For this review, take the finished solid that the model builds, in its own axes (mm). A direction names the side the tool comes from. Round coordinates to 2 decimals unless told otherwise and drop trailing zeros. Loops run counter-clockwise (first coordinate to the right, second up) from the corner with the lowest first, then second, coordinate; pieces in that order, holes last.
1. Clearance check with flat-ended pins moving along their axes: pin 1 Ø2 at (x, z) = (-67, 3.5) entering from +Y (3 decimals); pin 2 Ø0.8 at (x, z) = (-26.5, -7) entering from +Y; pin 3 Ø4 at (x, z) = (-44.5, 1.5) entering from -Y (3 decimals). State where each tip first meets the part, or that it passes through.
2. Tool access review of faces 4 (the flat face through (-65.25, -1, 1)), 5 (the flat face through (-53.7, -6.405, 6.7)), 6 (the flat face through (-29, -0.89, 5)): name each direction out of +Z, -Z, +X, -X, +Y, -Y from which nothing blocks a thin tool from reaching the whole face with its end or side.
3. Consider section A-A on x = -47. State the section outline as (y, z) points (3 decimals).
4. To check wall thickness, follow line 1 along X through (y, z) = (2.75, 0.5); line 2 along Z through (x, y) = (-40, -4.75); line 3 along Y through (x, z) = (-26.75, -6.9) (3 decimals). State the ranges of each line that lie inside material, in increasing order.
5. Consider section B-B on x = -59. State the section outline as (y, z) points (3 decimals).
6. Draft analysis for pull direction Z (two halves, no side actions). For faces 1 (the cylindrical face through (-73.087, -2.827, 6.014)), 2 (the flat face through (-29, 2, -6)), 3 (the flat face through (-70, 0, 5)), state which applies: released by +Z, released by -Z, zero draft, split by the parting line, or undercut.
Autodesk Inventor part; units mm, degrees
ref_plane "YZ Plane" through (0, 0, 0) normal (1, 0, 0) x (0, 1, 0)
ref_plane "XZ Plane" through (0, 0, 0) normal (0, 1, 0) x (-1, 0, 0)
ref_plane "XY Plane" through (0, 0, 0) normal (0, 0, 1) x (1, 0, 0)
ref_plane "Work Plane1" through (-21.75, 2.25, -0.6) normal (0, 0, 1) x (-1, 0, 0)
ref_plane "Work Plane2" through (-30.217, -5.375, 6) normal (0, 0, 1) x (1, 0, 0)
sketch "Sketch1" plane through (-30.217, -5.375, 6) normal (0, 0, 1) x (1, 0, 0)
  circle A0 centre (2.6155, -1.0303) radius 1.1
  circle A1 centre (3.467, 10) radius 1.5
  line L0 (4.6155, -1.0303) -> (5.967, 8)
  line L1 (0.6155, -1.0303) -> (-44.3845, -1.0303)
  arc A2 (0.6155, -1.0303) -> (4.6155, -1.0303) centre (2.6155, -1.0303) ccw
  line L2 (5.967, 8) -> (5.967, 10)
  line L3 (0.967, 10) -> (-44.033, 10)
  arc A3 (5.967, 10) -> (0.967, 10) centre (3.467, 10) ccw
  line L4 (-44.033, 10) -> (-44.3845, -1.0303)
  point P0 (30.217, 5.375)
  dimension "d0" = 2
  dimension "d1" = 2
  dimension "d2" = 2
  dimension "d3" = 2.5
  dimension "d4" = 2
  dimension "d5" = 2.5
  dimension "d6" = 2.5
  dimension "d7" = 45
  dimension "d8" = 45
extrude "Extrusion1" add sketch "Sketch1" along normal blind 1
sketch "Sketch2" plane through (-30.217, -5.375, 6) normal (0, 0, -1) x (-1, 0, 0)
  arc A0 (-0.967, 10) -> (-5.967, 10) centre (-3.467, 10) ccw
  line L0 (-5.967, 8) -> (-5.967, 10)
  line L1 (-4.6155, -1.0303) -> (-5.967, 8)
  arc A1 (-4.6155, -1.0303) -> (-0.6155, -1.0303) centre (-2.6155, -1.0303) ccw
  line L2 (44.3845, -1.0303) -> (-0.6155, -1.0303)
  line L3 (44.033, 10) -> (44.3845, -1.0303)
  line L4 (-0.967, 10) -> (44.033, 10)
  circle A2 centre (-2.6155, -1.0303) radius 1.1
  circle A3 centre (-3.467, 10) radius 1.5
  line L5 (44.3845, -1.0303) -> (-0.6155, -1.0303)
  line L6 (4.033, -1.0303) -> (4.033, 10)
  line L7 (-0.967, 10) -> (44.033, 10)
  point P0 (-30.217, 5.375)
  point P1 (4.033, 10)
  point P2 (4.033, -1.0303)
  dimension "d11" = 5
extrude "Extrusion2" add sketch "Sketch2" along normal blind 14 contours L4 L3 L2 L6
sketch "Sketch3" plane through (-30.217, -5.375, -8) normal (0, 0, -1) x (-1, 0, 0)
  circle A0 centre (-3.467, 10) radius 1.5
  line L0 (-8.467, 7.625) -> (-8.467, 12.375)
  line L1 (-8.467, 7.625) -> (-0.967, 7.625)
  line L2 (-0.967, 12.375) -> (-0.967, 7.625)
  line L3 (-8.467, 12.375) -> (-0.967, 12.375)
  line L4 (44.033, 10) -> (4.033, 10)
  line L5 (4.033, 10) -> (4.033, -1.0303)
  line L6 (4.033, -1.0303) -> (44.3845, -1.0303)
  line L7 (44.3845, -1.0303) -> (44.033, 10)
  circle A1 centre (-3.467, 10) radius 1.5
  circle A2 centre (-2.6155, -1.0303) radius 1.1
  line L8 (4.033, -1.0303) -> (4.033, 10)
  line L9 (-0.967, 10) -> (4.033, 10)
  arc A3 (-0.967, 10) -> (-5.967, 10) centre (-3.467, 10) ccw
  line L10 (-5.967, 8) -> (-5.967, 10)
  line L11 (-4.6155, -1.0303) -> (-5.967, 8)
  arc A4 (-4.6155, -1.0303) -> (-0.6155, -1.0303) centre (-2.6155, -1.0303) ccw
  line L12 (4.033, -1.0303) -> (-0.6155, -1.0303)
  line L13 (4.033, 10) -> (4.033, -1.0303)
  line L14 (4.033, 4.4849) -> (-5.4409, 4.4849)
  line L15 (-4.6155, -1.0303) -> (-5.967, 8)
  point P0 (-30.217, 5.375)
  point P1 (-5.4409, 4.4849)
  point P2 (-2.6863, 12.375)
  point P3 (-4.2476, 12.375)
extrude "Extrusion3" add sketch "Sketch3" against normal blind 2 contours L11 L10 A3 L3 L2 L1 | L1 L2 L9 L5 L14 L11
sketch "Sketch4" plane through (-30.217, -5.375, 6) normal (0, 0, -1) x (-1, 0, 0)
  circle A0 centre (-3.467, 10) radius 1.5
  circle A1 centre (-2.6155, -1.0303) radius 1.1
  line L0 (4.033, -1.0303) -> (4.033, 10)
  line L1 (-0.967, 10) -> (4.033, 10)
  arc A2 (-0.967, 10) -> (-5.967, 10) centre (-3.467, 10) ccw
  line L2 (-5.967, 8) -> (-5.967, 10)
  line L3 (-4.6155, -1.0303) -> (-5.967, 8)
  arc A3 (-4.6155, -1.0303) -> (-0.6155, -1.0303) centre (-2.6155, -1.0303) ccw
  line L4 (4.033, -1.0303) -> (-0.6155, -1.0303)
  circle A4 centre (-3.467, 10) radius 1.5
  circle A5 centre (-3.467, 10) radius 2.5
  arc A6 (-0.967, 10) -> (-5.967, 10) centre (-3.467, 10) ccw
  circle A7 centre (-3.467, 10) radius 1.5
  line L5 (44.033, 10) -> (-0.967, 10)
  arc A8 (-0.967, 10) -> (-2.6863, 12.375) centre (-3.467, 10) ccw
  line L6 (-2.6863, 12.375) -> (-4.2476, 12.375)
  arc A9 (-4.2476, 12.375) -> (-5.967, 10) centre (-3.467, 10) ccw
  line L7 (-5.967, 10) -> (-5.967, 8)
  line L8 (-5.967, 8) -> (-5.4409, 4.4849)
  line L9 (-5.4409, 4.4849) -> (4.033, 4.4849)
  line L10 (4.033, 4.4849) -> (4.033, -1.0303)
  line L11 (4.033, -1.0303) -> (44.3845, -1.0303)
  line L12 (44.3845, -1.0303) -> (44.033, 10)
  point P0 (-30.217, 5.375)
extrude "Extrusion4" add sketch "Sketch4" along normal blind 2 contours L9 L3 L2 A5 L1 L0 | A5 A2 L6
sketch "Sketch5" plane through (-74.25, 4.625, 7) normal (0, 1, 0) x (1, 0, 0)
  line L0 (45, 3) -> (45, 0)
  line L1 (40, 3) -> (45, 3)
  line L2 (40, 3) -> (40, 13)
  line L3 (45, 13) -> (40, 13)
  line L4 (45, 15) -> (45, 13)
  line L5 (0, 15) -> (45, 15)
  line L6 (0, 15) -> (0, 0)
  line L7 (45, 0) -> (0, 0)
  line L8 (8, 13) -> (-0.5, 13)
  line L9 (-0.5, 13) -> (-0.5, 2)
  line L10 (-0.5, 2) -> (8, 2)
  line L11 (8, 2) -> (8, 13)
  point P0 (74.25, 7)
  point P1 (8, 7.5)
  point P2 (0, 7.5)
  dimension "d18" = 8
  dimension "d19" = 0.5
  dimension "d20" = 2
extrude "Extrusion5" cut sketch "Sketch5" against normal blind 9 contours L10 L9 L8 L6 | L6 L8 L11 L10
shell "Shell1" thickness 1 removed faces 1 at (-61.1509, -6.4053, 1.6667)
sketch "Sketch6" plane through (-30.217, -5.375, 7) normal (0, 0, 1) x (1, 0, 0)
  circle A0 centre (-41.7707, 2.5) radius 1.1
  line L0 (-44.033, 10) -> (-44.3845, -1.0303) construction
  point P0 (30.217, 5.375)
  point P1 (-44.3198, 1)
  dimension "d24" = 2.2
  dimension "d25" = 1.5
  dimension "d26" = 2.5
extrude "Extrusion6" cut sketch "Sketch6" against normal up to surface (2 mm away)
sketch "Sketch7" plane through (-30.217, -5.375, 7) normal (0, 0, 1) x (1, 0, 0)
  circle A0 centre (-41.5955, 8) radius 1.1
  circle A1 centre (-41.7707, 2.5) radius 1.1 construction
  line L0 (-44.033, 10) -> (-44.3845, -1.0303) construction
  line L1 (0.967, 10) -> (-44.033, 10) construction
  point P0 (30.217, 5.375)
  dimension "d29" = 2.2
  dimension "d30" = 2.5
  dimension "d31" = 2
extrude "Extrusion7" cut sketch "Sketch7" against normal up to surface (2 mm away)
sketch "Sketch8" plane through (-74.25, 4.625, 7) normal (0, 1, 0) x (1, 0, 0)
  line L0 (0, 13) -> (8, 13)
  line L1 (8, 13) -> (8, 2)
  line L2 (8, 2) -> (0, 2)
  line L3 (0, 2) -> (0, 0)
  line L4 (45, 0) -> (0, 0)
  line L5 (45, 3) -> (45, 0)
  line L6 (40, 3) -> (45, 3)
  line L7 (40, 3) -> (40, 13)
  line L8 (45, 13) -> (40, 13)
  line L9 (45, 15) -> (45, 13)
  line L10 (0, 15) -> (45, 15)
  line L11 (0, 15) -> (0, 13)
  line L12 (-0.2867, 2) -> (-0.2867, 13)
  line L13 (8, 2) -> (-0.2867, 2)
  line L14 (8, 13) -> (8, 2)
  line L15 (-0.2867, 13) -> (8, 13)
  line L16 (-0.3514, 15) -> (-0.3514, 0)
  line L17 (0, 15) -> (45, 15)
  arc A0 (-0.3514, 11) -> (25, 15) centre (-0.3514, 93.3367) ccw
  line L18 (-0.3514, 15) -> (0, 15)
  point P0 (74.25, 7)
  point P1 (25, 15)
  dimension "d34" = 20
  dimension "d35" = 4
extrude "Extrusion8" cut sketch "Sketch8" against normal up to next contours L11 L10 A0 L1 L0 | L15 L12 A0 L16 L18 L11 | L0 L1 A0 L12 L15
sketch "Sketch9" plane through (-30.217, -5.375, 7) normal (0, 0, 1) x (1, 0, 0)
  circle A0 centre (-41.5955, 8) radius 1.1
  circle A1 centre (-41.7707, 2.5) radius 1.1
  arc A2 (5.967, 10) -> (0.967, 10) centre (3.467, 10) ccw
  line L0 (0.967, 10) -> (-44.033, 10)
  line L1 (-44.033, 10) -> (-44.3845, -1.0303)
  line L2 (-44.3845, -1.0303) -> (0.6155, -1.0303)
  arc A3 (0.6155, -1.0303) -> (4.6155, -1.0303) centre (2.6155, -1.0303) ccw
  line L3 (4.6155, -1.0303) -> (5.967, 8)
  line L4 (5.967, 8) -> (5.967, 10)
  circle A4 centre (2.6155, -1.0303) radius 1.1
  circle A5 centre (3.467, 10) radius 1.5
  circle A6 centre (-38.0955, 8) radius 1.1
  point P0 (30.217, 5.375)
  dimension "d38" = 2.2
  dimension "d39" = 3.5
extrude "Extrusion9" cut sketch "Sketch9" against normal up to surface (2 mm away) contours A6
sketch "Sketch10" plane through (-30.217, -5.375, -8) normal (0, 0, -1) x (-1, 0, 0)
  circle A0 centre (-2.6155, -1.0303) radius 1.1 construction
  circle A1 centre (-3.467, 10) radius 1.5 construction
  circle A2 centre (-2.6155, -1.0303) radius 11.0631 construction
  point P0 (-30.217, 5.375)
properties part number "Dedo_1"
Resolved:
1. pin 1: stops at y = 4.625
1. pin 2: stops at y = 7
1. pin 3: stops at y = 3.625
2. face 4: -Z, -Y
2. face 5: +Z, -Z, -X, -Y
2. face 6: -Z, +X, -Y
3. outline: (-6.405, -8) - (4.625, -8) - (4.625, 7) - (-6.405, 7) - (-6.405, 6) - (3.625, 6) - (3.625, -7) - (-6.405, -7) - close
4. line 1: x = -66.25 to -65.25, -35.25 to -34.25
4. line 2: z = -8 to -7, 6 to 7
4. line 3: y = -0.89 to 3.125, 6.125 to 7
5. outline: (-6.405, 6) - (3.625, 6) - (3.625, -5.492) - (4.625, -5.492) - (4.625, 7) - (-6.405, 7) - close
6. face 1: zero draft
6. face 2: undercut
6. face 3: released by -Z
